Design review of the part shown in the three views and the two pictorial views. Dimensions are in mm from the part's minimum x, y and z. Coordinates: 2 decimals unless noted, no trailing zeros. Loops run counter-clockwise (first coordinate to the right, second up) from the corner with the lowest first, then second, coordinate; pieces in that order, holes last. Notation, with made-up numbers: (-0.75, -35.5) -> (51.25, -35.5) arc R24 ccw to (51.25, -22.5) -> close; hole circle Ø6 at (81, -10.75). An arc over 180 degrees is marked (long way). One line per item, written item: value.
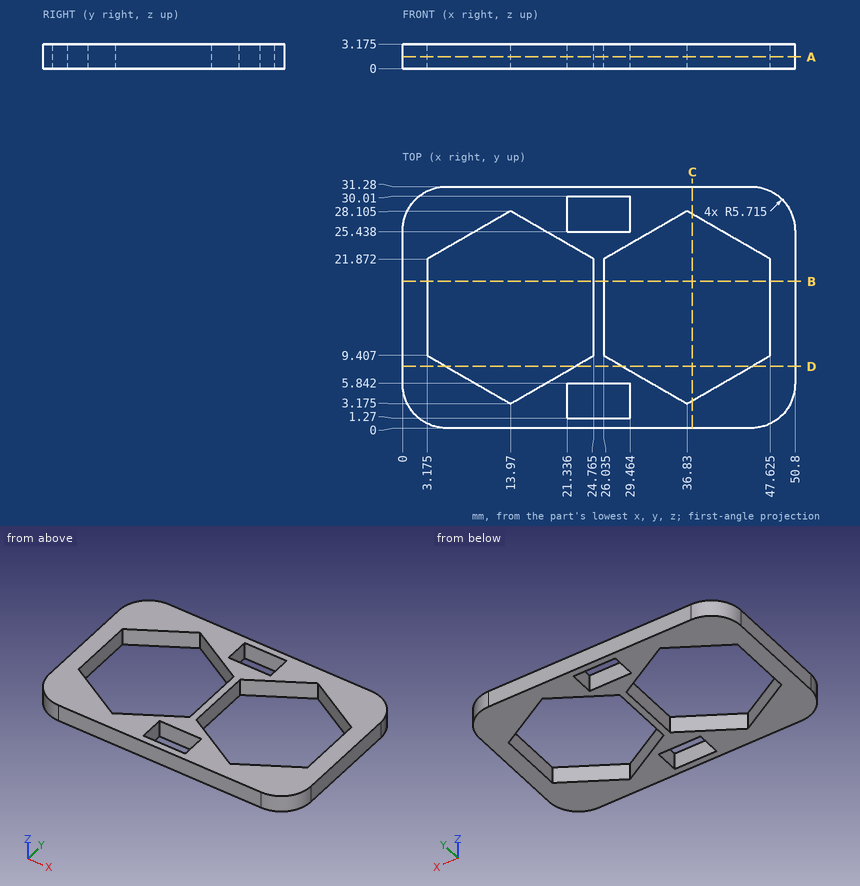
1. Insertion check: pin 1 Ø1 at (y, z) = (4.5, 2) entering from +X (1 decimal). The pin has a flat end and moves straight along its axis. Give the tip position at first contact, or say it passes through.
Return value:
pin 1: stops at x = 50.8
2. Take a section at B-B, the plane y = 19. Give the boundary of the cut face in (x, z) (1 decimal), and give its area (3 significant figures).
Return value:
outline: (0, 0) -> (3.2, 0) -> (3.2, 3.2) -> (0, 3.2) -> close; (24.8, 0) -> (26, 0) -> (26, 3.2) -> (24.8, 3.2) -> close; (47.6, 0) -> (50.8, 0) -> (50.8, 3.2) -> (47.6, 3.2) -> close
area: 24.2 mm2
3. Take a section at A-A, the plane z = 1.5. Give the boundary of the cut face in (x, y) (1 decimal).
Return value:
outline: (0, 5.7) arc R5.7 ccw to (5.7, 0) -> (45.1, 0) arc R5.7 ccw to (50.8, 5.7) -> (50.8, 25.6) arc R5.7 ccw to (45.1, 31.3) -> (5.7, 31.3) arc R5.7 ccw to (0, 25.6) -> close; hole (3.2, 9.4) -> (14, 3.2) -> (24.8, 9.4) -> (24.8, 21.9) -> (14, 28.1) -> (3.2, 21.9) -> close; hole (21.3, 1.3) -> (29.5, 1.3) -> (29.5, 5.8) -> (21.3, 5.8) -> close; hole (21.3, 25.4) -> (29.5, 25.4) -> (29.5, 30) -> (21.3, 30) -> close; hole (26, 9.4) -> (36.8, 3.2) -> (47.6, 9.4) -> (47.6, 21.9) -> (36.8, 28.1) -> (26, 21.9) -> close
4. To check wall thickness, follow probe 1 along X at (y, z) = (13.5, 0.95) (1 decimal); probe 2 along Y at (x, z) = (25.5, 3.05); probe 3 along X at (y, z) = (23, 2.6) (1 decimal). State the ranges of each line that lie inside material, in increasing order. Write a range as from..to.
Return value:
probe 1: x = 0..3.2, 24.8..26, 47.6..50.8
probe 2: y = 0..1.27, 5.84..25.44, 30.01..31.28
probe 3: x = 0..5.1, 22.8..28, 45.7..50.8
5. Take a section at C-C, the plane x = 37.5. Give the boundary of the cut face in (y, z) (1 decimal), and give its area (3 significant figures).
Return value:
outline: (0, 0) -> (3.6, 0) -> (3.6, 3.2) -> (0, 3.2) -> close; (27.7, 0) -> (31.3, 0) -> (31.3, 3.2) -> (27.7, 3.2) -> close
area: 22.6 mm2
6. Take a section at D-D, the plane y = 8. Give the boundary of the cut face in (x, z) (1 decimal).
Return value:
outline: (0, 0) -> (5.6, 0) -> (5.6, 3.2) -> (0, 3.2) -> close; (22.3, 0) -> (28.5, 0) -> (28.5, 3.2) -> (22.3, 3.2) -> close; (45.2, 0) -> (50.8, 0) -> (50.8, 3.2) -> (45.2, 3.2) -> close
